Work out the finished part from the listing and answer in its coordinate system (mm). Give positions to 0.01 mm unless a question says otherwise; leave off trailing zeros. Loops run counter-clockwise (first coordinate to the right, second up) from the corner with the lowest first, then second, coordinate; pieces in that order, holes last. Notation, with made-up numbers: (-9, 22.25) - (49, 22.25) arc R4 cw to (49, 27.25) - close; hole circle Ø5 at (-16, 34). An arc over 180 degrees is marked (long way). One line per item, written item: value.
from build123d import *

# Parameters (mm, degrees)
SKETCH_1_W          = 41
SKETCH_1_H          = 40
EXTRUDE_1_DEPTH     = 0.2
SKETCH_5_R          = 4.5
CUT_EXTRUDE_3_DEPTH = 0.2
SKETCH_6_R          = 1.5
CUT_EXTRUDE_4_DEPTH = 0.2
EXTRUDE_START       = 300
SKETCH_7_R          = 5.2
SKETCH_7_R_2        = 4.5
EXTRUDE_2_DEPTH     = 300


with BuildPart() as part:
    # 스케치1 → 보스-돌출1 (new body)
    with BuildSketch(Plane.XY):
        with Locations((20.5, 20)):
            Rectangle(SKETCH_1_W, SKETCH_1_H)
    extrude(amount=EXTRUDE_1_DEPTH)

    # 스케치5 → 컷-돌출3 (cut)
    with BuildSketch(Plane.XY.offset(0.2)):
        with Locations((20.7, 19.8)):
            Circle(SKETCH_5_R)
    extrude(amount=-CUT_EXTRUDE_3_DEPTH, mode=Mode.SUBTRACT)

    # 스케치6 → 컷-돌출4 (cut)
    with BuildSketch(Plane.XY.offset(0.2)):
        with Locations((20.7, 33.75)):
            Circle(SKETCH_6_R)
        with Locations((34.65, 33.75)):
            Circle(SKETCH_6_R)
        with Locations((34.65, 19.8)):
            Circle(SKETCH_6_R)
        with Locations((20.7, 5.85)):
            Circle(SKETCH_6_R)
        with Locations((34.65, 5.85)):
            Circle(SKETCH_6_R)
        with Locations((6.75, 5.85)):
            Circle(SKETCH_6_R)
        with Locations((6.75, 33.75)):
            Circle(SKETCH_6_R)
        with Locations((6.75, 19.8)):
            Circle(SKETCH_6_R)
    extrude(amount=-CUT_EXTRUDE_4_DEPTH, mode=Mode.SUBTRACT)

    # 스케치7 → 보스-돌출2 (add)
    with BuildSketch(Plane.XY.offset(0.2).offset(EXTRUDE_START)):
        with Locations((20.7, 19.8)):
            Circle(SKETCH_7_R)
        with Locations((20.7, 19.8)):
            Circle(SKETCH_7_R_2, mode=Mode.SUBTRACT)
    extrude(amount=-EXTRUDE_2_DEPTH)


solid = part.part
1. The mould has two halves that part along Y. Classify faces 1 (the cylindrical face through (23.099, 15.187, 152.3)), 2 (the flat face through (16, 25, 0.2)), 3 (the cylindrical face through (20.11, 24.26, 152.2)): released by +Y, released by -Y, zero draft, split by the parting line, or undercut.
Output:
face 1: split by the parting line
face 2: zero draft
face 3: undercut
2. Find the intervals of material crossed by line 1 along Y through (x, z) = (20.5, 15.5); line 2 along Y through (x, z) = (34.65, 0.1); line 3 along Z through (x, y) = (12.5, 14), in increasing order.
Output:
line 1: y = 14.6 to 15.3, 24.3 to 25
line 2: y = 0 to 4.35, 7.35 to 18.3, 21.3 to 32.25, 35.25 to 40
line 3: z = 0 to 0.2
3. Flat-ended cylindrical pins translate along their axes: pin 1 Ø12 at (x, z) = (16.5, 105) entering from -Y; pin 2 Ø5 at (x, y) = (20.7, 5.85) entering from -Z; pin 3 Ø5 at (x, z) = (26.5, 197.5) entering from +Y; pin 4 Ø1.5 at (x, y) = (12, 19.5) entering from +Z. Find the tip coordinate at first contact, or state that the pin passes through.
Output:
pin 1: stops at y = 14.6
pin 2: stops at z = 0
pin 3: stops at y = 23.82
pin 4: stops at z = 0.2
4. Section A-A (z = 226) is taken. Write down the section's boundary in (x, y).
Output:
outline: circle Ø10.4 at (20.7, 19.8); hole circle Ø9 at (20.7, 19.8)
